Input: part model. Units: mm. Frame: model coordinates. A direction names the side the tool comes from. Coordinates: 2 decimals unless noted, no trailing zeros. Write each loop counter-clockwise with the first axis right and the second up, starting at its lowest first coordinate (ties: lowest second). Pieces come first, ordered by that corner, then holes.
1) Draft query along X for faces 1 (the flat face through (66.5, 58, 0)), 2 (the flat face through (-4, -5, -4)), 3 (the flat face through (54, 40, 1)). Return one class per face: pulls with the +X half, pulls with the -X half, needs draft (parallel to the pull), parting line crosses it, or undercut.
2) Section query D-D (x = 18). Output: boundary loops of the cut face in (y, z), then the cut area to 3 significant figures.
3) Set-up query: faces 4 (the flat face through (64, 82, -27)), 5 (the flat face through (64, 109, 0)), 6 (the cylindrical face through (64.774, 75.272, 22.745)). Return all of +Z, -Z, +X, -X, +Y, -Y with unobstructed straight access to the full face (end or side cutting, diameter ignored); none if empty.
4) Section query A-A (y = 43). Output: boundary loops of the cut face in (x, z), then the cut area to 3 significant figures.
5) Section query C-C (z = 20). Output: boundary loops of the cut face in (x, y).
6) Pin query (flat end, axial travel): pin 1 Ø2 at (x, y) = (65, 63.5) entering from +Z; pin 2 Ø6.5 at (x, z) = (46, 35.02) entering from +Y; pin 3 Ø3 at (y, z) = (18, 25) entering from +X; pin 4 Ø16.5 at (x, z) = (0, 0) entering from -Y. Return the tip coordinate at first contact, or that it passes through.
7) Line query: L1, parallel to Y at x = 64.9, z = 24.5; L2, parallel to X at y = -4, z = 0 (3 decimals); L3, parallel to Y at x = 65, z = 24. Output: solid intervals per line, ascending.
8) Section query B-B (x = -46). Output: boundary loops of the cut face in (y, z).
from build123d import *

# Parameters (mm, degrees)
SKETCH_1_R           = 75
EXTRUDE_2_DEPTH      = 8
SKETCH_1_6_W         = 102
SKETCH_1_6_H         = 82
CUT_EXTRUDE_3_DEPTH  = 3
SKETCH_2_R           = 9.065
CUT_EXTRUDE_4_DEPTH  = 2
SKETCH_3_R           = 1.6
CUT_EXTRUDE_5_DEPTH  = 10
SKETCH_11_R          = 4.755489011
CUT_EXTRUDE_6_DEPTH  = 10
SKETCH_12_R          = 2.1
CUT_EXTRUDE_7_DEPTH  = 10
SKETCH_21_W          = 15.39960192
SKETCH_21_H          = 9.476678105
CUT_EXTRUDE_8_DEPTH  = 6
EXTRUDE_5_DEPTH      = 8
SKETCH_30_W          = 56
SKETCH_30_H          = 85
EXTRUDE_6_DEPTH      = 2.5
SKETCH_31_R          = 1.9
CUT_EXTRUDE_10_DEPTH = 3.5
FILLET_1_R           = 5
SKETCH_40_W          = 52
SKETCH_40_H          = 52
EXTRUDE_7_DEPTH      = 2
SKETCH_42_R          = 1.9
CUT_EXTRUDE_11_DEPTH = 3.5
SKETCH_52_R          = 2.1
CUT_EXTRUDE_12_DEPTH = 4


with BuildPart() as part:
    # Sketch 1 → Extrude 2 (new body)
    with BuildSketch(Plane(origin=(0, 0, 0), x_dir=(1, 0, 0), z_dir=(0, 1, 0))):
        with Locations(Location((0, 0, 0), (0, 0, 270))):
            Circle(SKETCH_1_R)
    extrude(amount=-EXTRUDE_2_DEPTH)

    # Sketch 1_6 → Cut-Extrude 3 (cut)
    with BuildSketch(Plane(origin=(0, 0, 0), x_dir=(1, 0, 0), z_dir=(0, 1, 0))):
        Rectangle(SKETCH_1_6_W, SKETCH_1_6_H)
    extrude(amount=-CUT_EXTRUDE_3_DEPTH, mode=Mode.SUBTRACT)

    # Sketch 2 → Cut-Extrude 4 (cut)
    with BuildSketch(Plane(origin=(0, -3, 0), x_dir=(1, 0, 0), z_dir=(0, 1, 0))):
        with Locations(Location((0, 0, 0), (0, 0, 270))):
            Circle(SKETCH_2_R)
    extrude(amount=-CUT_EXTRUDE_4_DEPTH, mode=Mode.SUBTRACT)

    # Sketch 3 → Cut-Extrude 5 (cut)
    with BuildSketch(Plane(origin=(0, -5, 0), x_dir=(1, 0, 0), z_dir=(0, 1, 0))):
        with Locations(Location((0, 6, 0), (0, 0, 270))):
            Circle(SKETCH_3_R)
        with Locations(Location((5.196152423, -3, 0), (0, 0, 270))):
            Circle(SKETCH_3_R)
        with Locations(Location((-5.196152423, -3, 0), (0, 0, 270))):
            Circle(SKETCH_3_R)
    extrude(amount=-CUT_EXTRUDE_5_DEPTH, mode=Mode.SUBTRACT)

    # Sketch 11 → Cut-Extrude 6 (cut)
    with BuildSketch(Plane(origin=(0, -5, 0), x_dir=(1, 0, 0), z_dir=(0, 1, 0))):
        Circle(SKETCH_11_R)
    extrude(amount=-CUT_EXTRUDE_6_DEPTH, mode=Mode.SUBTRACT)

    # Sketch 12 → Cut-Extrude 7 (cut)
    with BuildSketch(Plane(origin=(0, -3, 0), x_dir=(1, 0, 0), z_dir=(0, 1, 0))):
        with Locations(Location((-46, 36.980392157, 0), (0, 0, 270))):
            Circle(SKETCH_12_R)
        with Locations(Location((46, 36.980392157, 0), (0, 0, 270))):
            Circle(SKETCH_12_R)
        with Locations(Location((46, -35.019607843, 0), (0, 0, 270))):
            Circle(SKETCH_12_R)
        with Locations(Location((-46, -35.019607843, 0), (0, 0, 270))):
            Circle(SKETCH_12_R)
    extrude(amount=-CUT_EXTRUDE_7_DEPTH, mode=Mode.SUBTRACT)

    # Sketch 21 → Cut-Extrude 8 (cut)
    with BuildSketch(Plane(origin=(0, 0, 0), x_dir=(1, 0, 0), z_dir=(0, 1, 0))):
        with Locations((0, -44.066553185)):
            Rectangle(SKETCH_21_W, SKETCH_21_H)
    extrude(amount=-CUT_EXTRUDE_8_DEPTH, mode=Mode.SUBTRACT)

    # Sketch 24 → Extrude 5 (add)
    with BuildSketch(Plane.ZY.offset(-64)):
        with BuildLine():
            Line((-24, 100), (-30, 0))
            Line((-30, 0), (30, 0))
            Line((30, 0), (24, 100))
            ThreePointArc((24, 100), (0, 124), (-24, 100))
        make_face()
    extrude(amount=EXTRUDE_5_DEPTH)

    # Sketch 30 → Extrude 6 (add)
    with BuildSketch(Plane(origin=(64, 0, 0), x_dir=(0, 0, -1), z_dir=(1, 0, 0))):
        with Locations((0, 57.284476884)):
            Rectangle(SKETCH_30_W, SKETCH_30_H)
    extrude(amount=EXTRUDE_6_DEPTH)

    # Sketch 31 → Cut-Extrude 10 (cut)
    with BuildSketch(Plane(origin=(66.5, 0, 0), x_dir=(0, 0, -1), z_dir=(1, 0, 0))):
        with Locations((-24.5, 18)):
            Circle(SKETCH_31_R)
        with Locations((24.5, 18)):
            Circle(SKETCH_31_R)
        with Locations((24.5, 76)):
            Circle(SKETCH_31_R)
        with Locations((-24.5, 76)):
            Circle(SKETCH_31_R)
    extrude(amount=-CUT_EXTRUDE_10_DEPTH, mode=Mode.SUBTRACT)

    # Fillet 1
    fillet_1_edges = [part.edges().sort_by_distance(p)[0] for p in [
        (60, 0, -30),
        (60, 0, 30),
    ]]
    fillet(fillet_1_edges, radius=FILLET_1_R)

    # Sketch 40 → Extrude 7 (add)
    with BuildSketch(Plane.ZY.offset(-56)):
        with Locations((1, 40.006516634)):
            Rectangle(SKETCH_40_W, SKETCH_40_H)
    extrude(amount=EXTRUDE_7_DEPTH)

    # Sketch 42 → Cut-Extrude 11 (cut)
    with BuildSketch(Plane.ZY.offset(-54)):
        with Locations((-22.2, 63.206516634)):
            Circle(SKETCH_42_R)
        with Locations((24.2, 63.206516634)):
            Circle(SKETCH_42_R)
        with Locations((-22.2, 16.806516634)):
            Circle(SKETCH_42_R)
        with Locations((24.2, 16.806516634)):
            Circle(SKETCH_42_R)
    extrude(amount=-CUT_EXTRUDE_11_DEPTH, mode=Mode.SUBTRACT)

    # Sketch 52 → Cut-Extrude 12 (cut)
    with BuildSketch(Plane.ZY.offset(-56)):
        with Locations((10.606601718, 110.606601718)):
            Circle(SKETCH_52_R)
        with Locations((10.606601718, 89.393398282)):
            Circle(SKETCH_52_R)
        with Locations((-10.606601718, 89.393398282)):
            Circle(SKETCH_52_R)
        with Locations((-10.606601718, 110.606601718)):
            Circle(SKETCH_52_R)
    extrude(amount=-CUT_EXTRUDE_12_DEPTH, mode=Mode.SUBTRACT)


solid = part.part
Answer:
1. face 1: pulls with the +X half
1. face 2: undercut
1. face 3: pulls with the -X half
2. outline: (-8, -72.81) - (0, -72.81) - (0, -41) - (-3, -41) - (-3, 41) - (0, 41) - (0, 72.81) - (-8, 72.81) - close
2. area: 919 mm2
3. face 4: -Z, -X, +Y
3. face 5: +Z, -Z, +X, +Y
3. face 6: +X
4. outline: (54, -25) - (56, -25) - (56, -27.42) - (64, -27.42) - (64, -28) - (66.5, -28) - (66.5, 28) - (64, 28) - (64, 27.42) - (56, 27.42) - (56, 27) - (54, 27) - close
4. area: 683 mm2
5. outline: (-72.28, -8) - (72.28, -8) - (72.28, 0) - (64, 0) - (64, 14.78) - (66.5, 14.78) - (66.5, 99.78) - (64, 99.78) - (64, 113.27) - (56, 113.27) - (56, 66.01) - (54, 66.01) - (54, 14.01) - (56, 14.01) - (56, 0) - (51, 0) - (51, -3) - (-51, -3) - (-51, 0) - (-72.28, 0) - close
6. pin 1: stops at z = 28
6. pin 2: stops at y = -3
6. pin 3: stops at x = 66.5
6. pin 4: stops at y = -8
7. L1: y = -8 to 0, 14.78 to 16.1, 19.9 to 74.1, 77.9 to 99.78
7. L2: x = -75 to -9.065, 9.065 to 75
7. L3: y = -8 to 0, 14.78 to 16.17, 19.83 to 74.17, 77.83 to 99.78
8. outline: (-8, -59.24) - (0, -59.24) - (0, -41) - (-3, -41) - (-3, -39.08) - (-8, -39.08) - close; (-8, -34.88) - (-3, -34.88) - (-3, 32.92) - (-8, 32.92) - close; (-8, 37.12) - (-3, 37.12) - (-3, 41) - (0, 41) - (0, 59.24) - (-8, 59.24) - close
